from build123d import *

# Parameters (mm, degrees)
MAIN_BLOCK_DEPTH         = 90
MAIN_CUTOUT_DEPTH        = 10
MAIN_CUTOUT_DEPTH_BACK   = 72
TOP_SLOPE_CUT_DEPTH      = 12
TOP_SLOPE_CUT_DEPTH_BACK = 90
FIRST_STEP_CUT_DEPTH     = 90
SECOND_STEP_CUT_DEPTH    = 50
THIRD_STEP_CUT_DEPTH     = 20


with BuildPart() as part:
    # Sketch1 → Main Block (new body)
    with BuildSketch(Plane(origin=(0, 0, 0), x_dir=(1, 0, 0), z_dir=(0, 1, 0))):
        Polygon((0, 0), (0, 90), (72, 90), (72, 72), (54, -9.521656958), align=None)
    extrude(amount=MAIN_BLOCK_DEPTH)

    # Sketch4 → Main Cutout (cut, two sides)
    with BuildSketch(Plane.XY) as main_cutout_sk:
        Polygon((18, 40.5), (18, 22.5), (0, 18), (0, 90), (54, 90), (54, 67.5), (36, 63), (36, 45), align=None)
    extrude(amount=MAIN_CUTOUT_DEPTH, mode=Mode.SUBTRACT)
    extrude(main_cutout_sk.sketch, amount=-MAIN_CUTOUT_DEPTH_BACK, mode=Mode.SUBTRACT)

    # Sketch5 → Top Slope Cut (cut, two sides)
    with BuildSketch(Plane.XY) as top_slope_cut_sk:
        Polygon((0, 90), (72, 90), (0, 72), align=None)
    extrude(amount=TOP_SLOPE_CUT_DEPTH, mode=Mode.SUBTRACT)
    extrude(top_slope_cut_sk.sketch, amount=-TOP_SLOPE_CUT_DEPTH_BACK, mode=Mode.SUBTRACT)

    # Sketch6 → First Step Cut (cut)
    with BuildSketch(Plane(origin=(-4.235294118, 16.941176471, 0), x_dir=(-0.9701425, -0.242535625, 0), z_dir=(-0.242535625, 0.9701425, 0))):
        Polygon((-92.892158272, -2.856450573), (-85.203658571, 13.828337001), (-4.365641251, 0), (-4.365641251, -18), align=None)
    extrude(amount=FIRST_STEP_CUT_DEPTH, mode=Mode.SUBTRACT)

    # Sketch7 → Second Step Cut (cut)
    with BuildSketch(Plane(origin=(-8.470588235, 33.882352941, 0), x_dir=(-0.9701425, -0.242535625, 0), z_dir=(-0.242535625, 0.9701425, 0))):
        Polygon((-27.285257817, -14.079317723), (-101.742779454, -1.342442975), (-101.770582014, -19.337687006), (-27.285257817, -32.079317723), align=None)
    extrude(amount=SECOND_STEP_CUT_DEPTH, mode=Mode.SUBTRACT)

    # Sketch8 → Third Step Cut (cut)
    with BuildSketch(Plane(origin=(-12.705882353, 50.823529412, 0), x_dir=(-0.9701425, -0.242535625, 0), z_dir=(-0.242535625, 0.9701425, 0))):
        Polygon((-50.204874383, -28.158635446), (-102.913338561, -19.142204445), (-106.827474424, -36.47264337), (-50.204874383, -46.158635446), align=None)
    extrude(amount=THIRD_STEP_CUT_DEPTH, mode=Mode.SUBTRACT)


solid = part.part
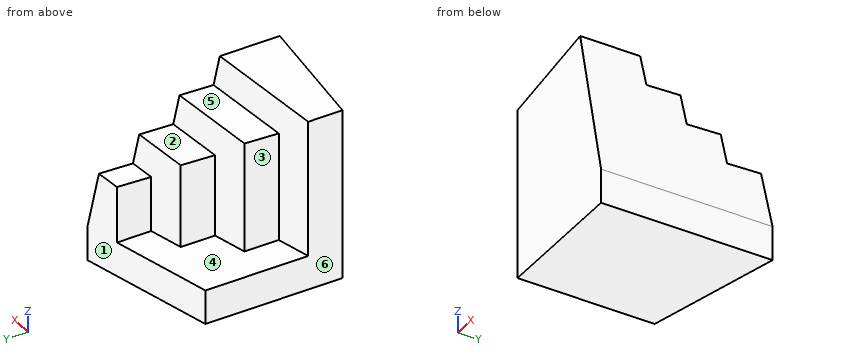
Build history of the part. All positions in model axes, mm. Face numbers are marked on the shaded views. A direction names the side the tool comes from. Give positions to 0.01 mm unless a question says otherwise; leave off trailing zeros. Order: outer loops, then holes, each group sorted by start corner. A loop starts at its lowest first (then second) coordinate and runs counter-clockwise, first axis right, second up. Notation, with made-up numbers: M -19.75,63 L 10.25,63 A35 ccw 10.25,98 Z; hole C -30.5,26 d5. An arc over 180 degrees is marked long. Put each result on its own line as item: value.
Item 1: Two-plate mould, pull along Y, no slides. Class the marked faces 1, 2 and 3: +Y half, -Y half, draft (parallel to the pull), parting line (faces both ways), or undercut.
From the geometry:
face 1: +Y half
face 2: undercut
face 3: draft
Item 2: Slice it at A-A, the plane y = 57.5. Write the cut outline in (x, z).
From the geometry:
outline: M 0,-90 L 72,-90 L 72,-72 L 61.44,-24.17 L 36,-28.39 L 36,-72 L 0,-72 Z
Item 3: 3-axis set-ups, long thin cutter, end or side, ignore diameter. For the marked faces 4, 5 and 6: which of +Z, -Z, +X, -X, +Y, -Y reach the whole face in a straight line?
From the geometry:
face 4: +Z, -X, +Y
face 5: +Z, -X
face 6: +Z, -Z, -X, +Y, -Y
Item 4: Flat gauge pins, fed straight in: pin 1 Ø2 at (y, z) = (46.5, -34) entering from -X; pin 2 Ø2 at (y, z) = (77, -49.5) entering from +X; pin 3 Ø8 at (x, z) = (18.5, -13) entering from +Y. Where does each tip first touch, or does it go through?
From the geometry:
pin 1: stops at x = 36
pin 2: stops at x = 67.25
pin 3: stops at y = 41.62
Item 5: Probe line 1 (Z direction, x = 22, y = 74.5); line 2 (Z direction, x = 18.5, y = 17); line 3 (Y direction, x = 15.5, z = -57) (3 decimals). List the from-to ranges inside material, lowest first. Write a range as [from, to].
From the geometry:
line 1: z = [-90, -72]
line 2: z = [-90, 3.26]
line 3: y = [0, 21.875]
Item 6: Slice it at C-C, the plane z = -56. Write the cut outline in (x, y).
From the geometry:
outline: M 0,0 L 68.47,0 L 68.47,89.12 L 54,85.5 L 54,67.5 L 36,63 L 36,45 L 18,40.5 L 18,22.5 L 0,18 Z
Item 7: Slice it at D-D, the plane y = 34. Write the cut outline in (x, z).
From the geometry:
outline: M 0,-90 L 72,-90 L 72,-72 L 57.81,-7.74 L 18,-14.35 L 18,-72 L 0,-72 Z
Item 8: Slice it at B-B, the plane x = 46. Write the cut outline in (y, z).
From the geometry:
outline: M 0,-90 L 83.5,-90 L 83.5,-72 L 65.5,-72 L 65.5,-26.4 L 47.5,-27.14 L 47.5,-9.14 L 29.5,-9.89 L 29.5,8.11 L 0,8.11 Z
